```python
from build123d import *

# Parameters (mm, degrees)
SKETCH1_W           = 79
SKETCH1_H           = 52
SKETCH1_W_2         = 75
SKETCH1_H_2         = 48
BOSS_EXTRUDE1_DEPTH = 4.524
SKETCH2_W           = 79
SKETCH2_H           = 52
BOSS_EXTRUDE2_DEPTH = 2
SKETCH3_R           = 1.9
CUT_EXTRUDE1_DEPTH  = 2
SKETCH4_R           = 2.75
SKETCH4_R_2         = 1.75
BOSS_EXTRUDE3_DEPTH = 3


with BuildPart() as part:
    # Sketch1 → Boss-Extrude1 (new body)
    with BuildSketch(Plane(origin=(0, 0, 0), x_dir=(1, 0, 0), z_dir=(0, 1, 0))):
        Rectangle(SKETCH1_W, SKETCH1_H)
        Rectangle(SKETCH1_W_2, SKETCH1_H_2, mode=Mode.SUBTRACT)
    extrude(amount=BOSS_EXTRUDE1_DEPTH)

    # Sketch2 → Boss-Extrude2 (add)
    with BuildSketch(Plane.XZ):
        Rectangle(SKETCH2_W, SKETCH2_H)
    extrude(amount=BOSS_EXTRUDE2_DEPTH)

    # Sketch3 → Cut-Extrude1 (cut)
    with BuildSketch(Plane(origin=(0, 0, 0), x_dir=(1, 0, 0), z_dir=(0, 1, 0))):
        with Locations(Location((-34, 20.5, 0), (0, 0, 270))):
            Circle(SKETCH3_R)
        with Locations(Location((34, 20.5, 0), (0, 0, 270))):
            Circle(SKETCH3_R)
        with Locations(Location((34, -20.5, 0), (0, 0, 270))):
            Circle(SKETCH3_R)
        with Locations(Location((-34, -20.5, 0), (0, 0, 270))):
            Circle(SKETCH3_R)
    extrude(amount=-CUT_EXTRUDE1_DEPTH, mode=Mode.SUBTRACT)

    # Sketch4 → Boss-Extrude3 (add)
    # profile 1 of 4: a face of its own
    with BuildSketch(Plane(origin=(0, 0, 0), x_dir=(1, 0, 0), z_dir=(0, 1, 0))):
        with Locations(Location((-34, -20.5, 0), (0, 0, 270))):
            Circle(SKETCH4_R)
        with Locations(Location((-34, -20.5, 0), (0, 0, 270))):
            Circle(SKETCH4_R_2, mode=Mode.SUBTRACT)
    # profile 2 of 4: a face of its own
    with BuildSketch(Plane(origin=(0, 0, 0), x_dir=(1, 0, 0), z_dir=(0, 1, 0))):
        with Locations(Location((34, -20.5, 0), (0, 0, 270))):
            Circle(SKETCH4_R)
        with Locations(Location((34, -20.5, 0), (0, 0, 270))):
            Circle(SKETCH4_R_2, mode=Mode.SUBTRACT)
    # profile 3 of 4: a face of its own
    with BuildSketch(Plane(origin=(0, 0, 0), x_dir=(1, 0, 0), z_dir=(0, 1, 0))):
        with Locations(Location((34, 20.5, 0), (0, 0, 270))):
            Circle(SKETCH4_R)
        with Locations(Location((34, 20.5, 0), (0, 0, 270))):
            Circle(SKETCH4_R_2, mode=Mode.SUBTRACT)
    # profile 4 of 4: a face of its own
    with BuildSketch(Plane(origin=(0, 0, 0), x_dir=(1, 0, 0), z_dir=(0, 1, 0))):
        with Locations(Location((-34, 20.5, 0), (0, 0, 270))):
            Circle(SKETCH4_R)
        with Locations(Location((-34, 20.5, 0), (0, 0, 270))):
            Circle(SKETCH4_R_2, mode=Mode.SUBTRACT)
    extrude(amount=BOSS_EXTRUDE3_DEPTH)


solid = part.part
```
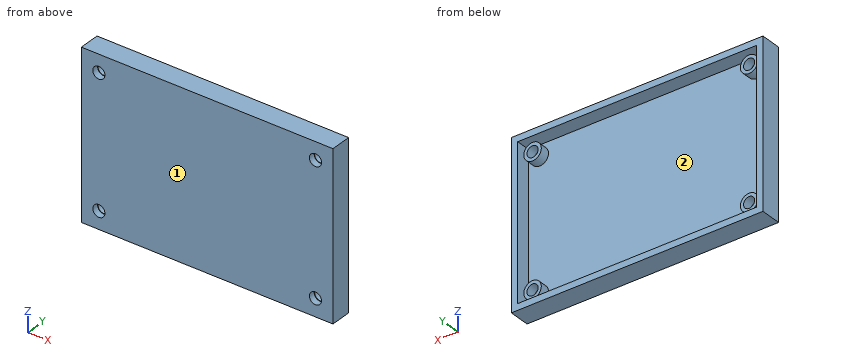
Check sheet for the modelled part. Datum: model origin and axes. Units: mm. Face numbers are marked on the shaded views. Round coordinates to 2 decimals unless told otherwise and drop trailing zeros. Order: outer loops, then holes, each group sorted by start corner. A loop starts at its lowest first (then second) coordinate and runs counter-clockwise, first axis right, second up. Notation, with made-up numbers: (-32, 35) -> (-24, 35) arc R18 ccw to (-24, 67) -> close; hole circle Ø1 at (5.25, 1.25). An arc over 180 degrees is marked (long way). One line per item, written item: value. Start each with the question number.
Q1. Cross-section at A-A (y = 1.5). Give the number of separate pieces and of enclosed holes in the cut face, and give its area (3 significant figures).
Q2. Cross-section at D-D (z = 11). Record the boundary of the cut face in (x, y), and give its area (3 significant figures).
Q3. Gauge pin test, flat ends, axial feed: pin 1 Ø1.6 at (x, z) = (-34, -21) entering from +Y; pin 2 Ø6 at (x, z) = (33.5, 20.5) entering from +Y. Record the tip position at first contact, or that the pin passes through.
Q4. Mould release check, pull along Z, two halves, no side actions. Record for the marked faces 1 and 2: pulls with the +Z half, pulls with the -Z half, needs draft (parallel to the pull), parting line crosses it, or undercut.
Q5. Thickness scan on line 1 (X direction, y = 1.2, z = -20.5); line 2 (Z direction, x = 10, y = 1); line 3 (X direction, y = -1.25, z = -20.5). Record the ranges inside material, lowest first.
Completed:
1. separate pieces: 5
1. enclosed holes: 5
1. area: 565 mm²
2. outline: (-39.5, -2) -> (39.5, -2) -> (39.5, 4.52) -> (37.5, 4.52) -> (37.5, 0) -> (-37.5, 0) -> (-37.5, 4.52) -> (-39.5, 4.52) -> close
2. area: 176 mm²
3. pin 1: passes through
3. pin 2: stops at y = 3
4. face 1: needs draft
4. face 2: undercut
5. line 1: x = -39.5 to -37.5, -36.75 to -35.75, -32.25 to -31.25, 31.25 to 32.25, 35.75 to 36.75, 37.5 to 39.5
5. line 2: z = -26 to -24, 24 to 26
5. line 3: x = -39.5 to -35.9, -32.1 to 32.1, 35.9 to 39.5
